Part print with two shaded views. Sizes in mm from the minimum x, y, z corner. Round coordinates to 2 decimals unless told otherwise and drop trailing zeros. Write each loop counter-clockwise with the first axis right and the second up, starting at its lowest first coordinate (ties: lowest second). Pieces come first, ordered by that corner, then holes. Notation, with made-up numbers: M -24.5,60.25 L 27.5,60.25 A11 cw 27.5,79.25 Z; hole C 62,-22.5 d4. An arc over 180 degrees is marked long. Use one line per item in the form item = value. Start each with the question number.
Item 1: Flat gauge pins, fed straight in: pin 1 Ø4 at (x, y) = (288.5, 9) entering from +Z; pin 2 Ø3 at (x, y) = (211.5, 6.5) entering from +Z. Where does each tip first touch, or does it go through?
Item 2: Probe L1, parallel to X at y = 9.5, z = 815; L2, parallel to Z at x = 232.5, y = 9.25. List the from-to ranges inside material, lowest first.
Item 3: Cut at A-A, the plane y = 6.25. Give the cut face in (x, z) (3 decimals).
Item 4: Cut at B-B, the plane x = 297. Give the cut face in (y, z).
Item 5: Cut at C-C, the plane x = 145. Give the cut face in (y, z).
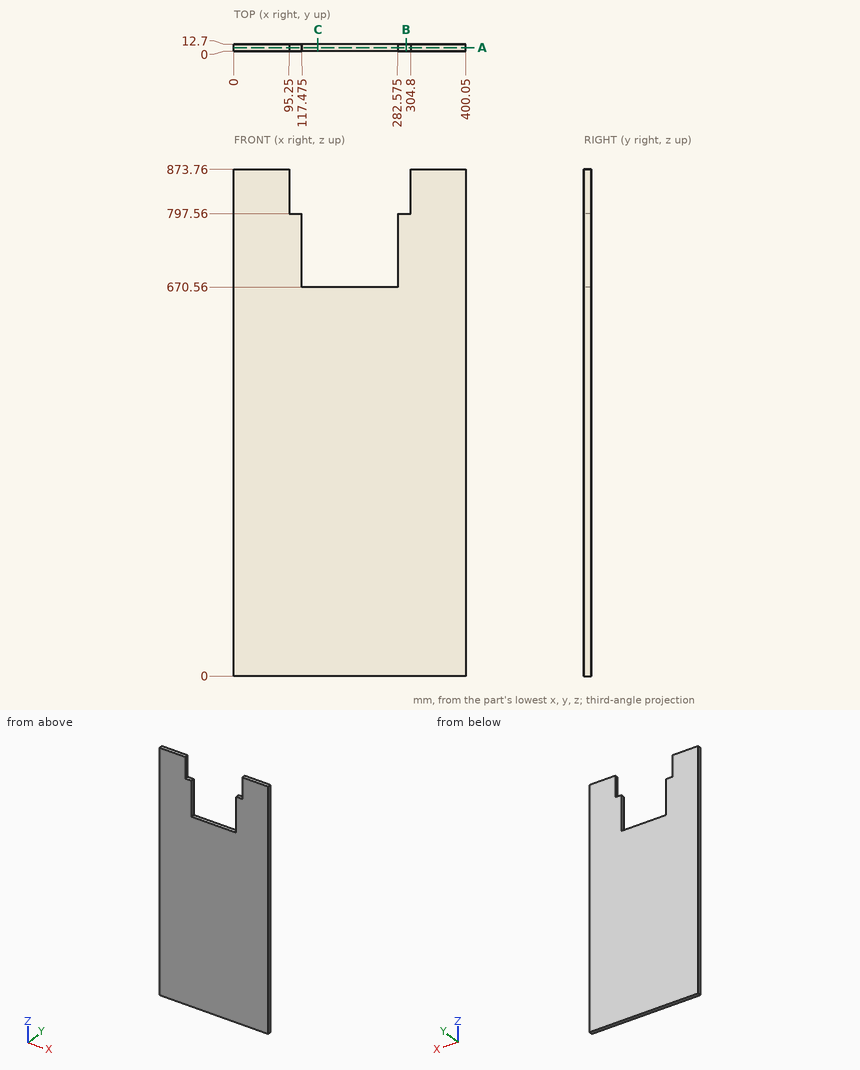
Model answer:
q1.pin_1 = 797.56
q1.pin_2 = 670.56
q2.L1 = 0 to 95.25, 304.8 to 400.05
q2.L2 = 0 to 670.56
q3.outline = M 0,0 L 400.05,0 L 400.05,873.76 L 304.8,873.76 L 304.8,797.56 L 282.575,797.56 L 282.575,670.56 L 117.475,670.56 L 117.475,797.56 L 95.25,797.56 L 95.25,873.76 L 0,873.76 Z
q4.outline = M 0,0 L 12.7,0 L 12.7,797.56 L 0,797.56 Z
q5.outline = M 0,0 L 12.7,0 L 12.7,670.56 L 0,670.56 Z
